Could you check a few things on this model? Use its own coordinates, in mm. Face numbers are marked on the shaded views. A direction names the side the tool comes from. Coordinates: 2 decimals unless noted, no trailing zeros. Loops run counter-clockwise (first coordinate to the right, second up) from the corner with the lowest first, then second, coordinate; pieces in that order, holes last. Notation, with made-up numbers: (81.25, -5) - (123.25, -5) arc R29 cw to (123.25, 25) - close; hole circle Ø2 at (48, 22). An arc over 180 degrees is marked (long way). One line per question, with ' | ' between items. Start each with the question number.
1. Please list where these lines run through material, in increasing order: L1, parallel to Z at x = 0.85, y = 1.7; L2, parallel to Z at x = 0.25, y = -0.2; L3, parallel to Y at x = -0.55, z = -4.5. Write a range as [from, to].
2. I want a section at A-A, the plane y = 0. Write out the boundary of the cut face in (x, z).
3. Which directions (+Z, -Z, +X, -X, +Y, -Y) give clear straight access to the entire face, cutting with the end or side of a thin tool? Please do the marked faces 1 and 2.
4. I'm going to push flat-ended pins straight in: P1, Ø1.1, axis at y = 1, z = 1.5, coming from the +X side; P2, Ø2, axis at x = 1, z = -9.5, coming from the -Y side; P3, Ø0.5, axis at x = 1, z = 1.5, coming from the -Y side. Where does each tip first touch, or does it pass through?
5. I want a section at B-B, the plane x = 0.6. Write out the boundary of the cut face in (y, z).
6. I want a section at C-C, the plane z = -4.75. Write out the boundary of the cut face in (x, y).
from build123d import *

# Parameters (mm, degrees)
SKETCH1_R           = 2
BOSS_EXTRUDE1_DEPTH = 2
SKETCH2_R           = 1.5
BOSS_EXTRUDE2_DEPTH = 15
SKETCH4_W           = 0.5
SKETCH4_H           = 1.25
SKETCH4_H_2         = 0.5
SKETCH4_W_2         = 1.25
CUT_EXTRUDE1_DEPTH  = 1


with BuildPart() as part:
    # Sketch1 → Boss-Extrude1 (new body)
    with BuildSketch(Plane.XY):
        Circle(SKETCH1_R)
    extrude(amount=BOSS_EXTRUDE1_DEPTH)

    # Sketch2 → Boss-Extrude2 (add)
    with BuildSketch(Plane(origin=(0, 0, 0), x_dir=(-1, 0, 0), z_dir=(0, 0, -1))):
        Circle(SKETCH2_R)
    extrude(amount=BOSS_EXTRUDE2_DEPTH)

    # Sketch4 → Cut-Extrude1 (cut)
    with BuildSketch(Plane.XY.offset(2)):
        with Locations((0, 0.875)):
            Rectangle(SKETCH4_W, SKETCH4_H)
        Rectangle(SKETCH4_W, SKETCH4_H_2)
        with Locations((0.875, 0)):
            Rectangle(SKETCH4_W_2, SKETCH4_H_2)
        with Locations((0, -0.875)):
            Rectangle(SKETCH4_W, SKETCH4_H)
        with Locations((-0.875, 0)):
            Rectangle(SKETCH4_W_2, SKETCH4_H_2)
    extrude(amount=-CUT_EXTRUDE1_DEPTH, mode=Mode.SUBTRACT)


solid = part.part
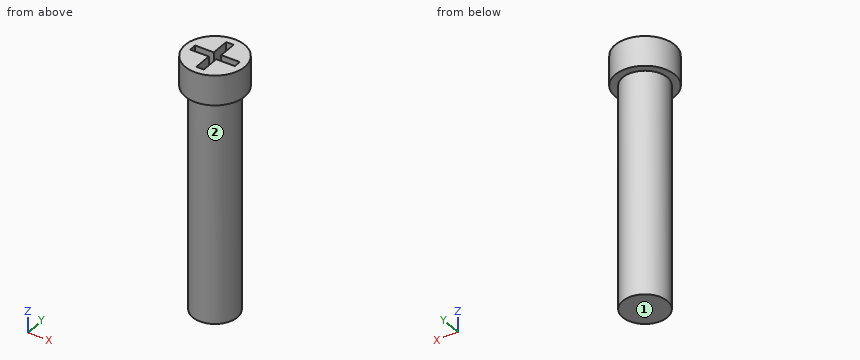
Results are:
1) L1: z = [0, 2] | L2: z = [-15, 1] | L3: y = [-1.4, 1.4]
2) outline: (-2, 0) - (-1.5, 0) - (-1.5, -15) - (1.5, -15) - (1.5, 0) - (2, 0) - (2, 2) - (1.5, 2) - (1.5, 1) - (-1.5, 1) - (-1.5, 2) - (-2, 2) - close
3) face 1: -Z, +X, -X, +Y, -Y | face 2: -Z
4) P1: stops at x = 1.95 | P2: stops at y = -1.5 | P3: stops at y = -1.85
5) outline: (-1.91, 0) - (-1.37, 0) - (-1.37, -15) - (1.37, -15) - (1.37, 0) - (1.91, 0) - (1.91, 2) - (0.25, 2) - (0.25, 1) - (-0.25, 1) - (-0.25, 2) - (-1.91, 2) - close
6) outline: circle Ø3 at (0, 0)
